Model file for the job. Use its own axes, mm. Round coordinates to 2 decimals unless told otherwise and drop trailing zeros. Write each loop counter-clockwise with the first axis right and the second up, starting at its lowest first coordinate (ties: lowest second). Pieces come first, ordered by that corner, then holes. Notation, with made-up numbers: (-10, 78) - (3, 78) arc R18 cw to (3, 84) - close; hole circle Ø11 at (-36, 59). An arc over 180 degrees is marked (long way). One line per item, written item: value.
from build123d import *

# Parameters (mm, degrees)
BOSS_EXTRUDE1_DEPTH     = 150
BOSS_EXTRUDE6_DEPTH     = 1.5
SKETCH7_R               = 0.5
CUT_EXTRUDE1_DEPTH      = 8.5
CUT_EXTRUDE1_DEPTH_BACK = 8.5
SKETCH9_R               = 0.5
CUT_EXTRUDE2_DEPTH      = 10


with BuildPart() as part:
    # Sketch1 → Boss-Extrude1 (new body)
    with BuildSketch(Plane.XY):
        with BuildLine():
            Line((7.5, 5), (5, 5))
            ThreePointArc((5, 5), (0, 0), (-5, 5))
            Line((-5, 5), (-7.5, 5))
            Line((-7.5, 5), (-7.5, -5))
            Line((-7.5, -5), (7.5, -5))
            Line((7.5, -5), (7.5, 5))
        make_face()
    extrude(amount=BOSS_EXTRUDE1_DEPTH)

    # Sketch6 → Boss-Extrude6 (add, symmetric)
    with BuildSketch(Plane.ZY):
        with BuildLine():
            ThreePointArc((77.5, -8), (75, -5.5), (72.5, -8))
            Line((72.5, -8), (77.5, -8))
        make_face()
        with BuildLine():
            Line((77.5, -8), (72.5, -8))
            ThreePointArc((72.5, -8), (75, -10.5), (77.5, -8))
        make_face()
        with BuildLine():
            Line((77.5, -5), (72.5, -5))
            Line((72.5, -5), (72.5, -8))
            ThreePointArc((72.5, -8), (75, -5.5), (77.5, -8))
            Line((77.5, -8), (77.5, -5))
        make_face()
    boss_extrude6 = extrude(amount=BOSS_EXTRUDE6_DEPTH, both=True)

    # Mirror1: Boss-Extrude6 across plane
    add(boss_extrude6.mirror(Plane(origin=(0, 0, 45), x_dir=(1, 0, 0), z_dir=(0, 0, -1))))

    # Sketch7 → Cut-Extrude1 (cut, two sides)
    with BuildSketch(Plane.ZY) as cut_extrude1_sk:
        with Locations((75, -8)):
            Circle(SKETCH7_R)
    extrude(amount=CUT_EXTRUDE1_DEPTH, mode=Mode.SUBTRACT)
    extrude(cut_extrude1_sk.sketch, amount=-CUT_EXTRUDE1_DEPTH_BACK, mode=Mode.SUBTRACT)

    # Sketch9 → Cut-Extrude2 (cut)
    with BuildSketch(Plane.ZY.offset(1.5)):
        with Locations((15, -8)):
            Circle(SKETCH9_R)
    extrude(amount=-CUT_EXTRUDE2_DEPTH, mode=Mode.SUBTRACT)


solid = part.part
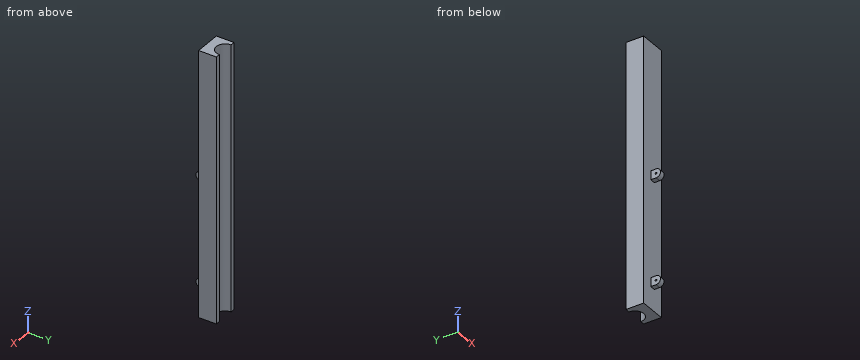
1. Band-saw the part on C-C on y = 2.75. Write the cut outline in (x, z), plus the area to 3 significant figures.
Report:
outline: (-7.5, 0) - (-4.47, 0) - (-4.47, 150) - (-7.5, 150) - close; (4.47, 0) - (7.5, 0) - (7.5, 150) - (4.47, 150) - close
area: 910 mm²
2. Wall check: probe 1 along Y at (x, z) = (0.3, 15); probe 2 along X at (y, z) = (1.5, 130); probe 3 along Y at (x, z) = (0, 19.5). Give the ranges that are in metal, low to high. Write a range as [from, to].
Report:
probe 1: [-10.5, -8.5], [-7.5, 0.01]
probe 2: [-7.5, -3.57], [3.57, 7.5]
probe 3: [-5, 0]
3. Drop flat-ended pins along their axis: pin 1 (4 mm diameter, centred on x = 2.5, z = 104, fed in from -Y); pin 2 (4 mm diameter, centred on y = -9, z = 15.5, fed in from +X); pin 3 (5.5 mm diameter, centred on y = -8, z = 74.5, fed in from -X); pin 4 (1 mm diameter, centred on x = -3, y = -6.5, fed in from +Z) (1 decimal). Give the stop position or say it passes through.
Report:
pin 1: y = -5
pin 2: x = 1.5
pin 3: x = -1.5
pin 4: through
4. Band-saw the part on B-B on z = 110. Write the cut outline in (x, y).
Report:
outline: (-7.5, -5) - (7.5, -5) - (7.5, 5) - (5, 5) arc R5 cw to (-5, 5) - (-7.5, 5) - close
5. Band-saw the part on A-A on y = -6.25. Write the cut outline in (x, z), plus the area to 3 significant figures.
Report:
outline: (-1.5, 12.5) - (1.5, 12.5) - (1.5, 17.5) - (-1.5, 17.5) - close; (-1.5, 72.5) - (1.5, 72.5) - (1.5, 77.5) - (-1.5, 77.5) - close
area: 30.0 mm²
6. Band-saw the part on D-D on x = 3.75. Write the cut outline in (y, z).
Report:
outline: (-5, 0) - (1.69, 0) - (1.69, 150) - (-5, 150) - close
